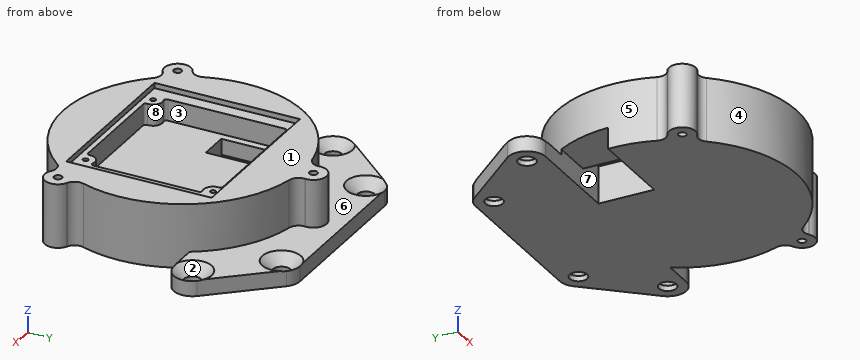
```python
from build123d import *

# Parameters (mm, degrees)
SKETCH_1_R                       = 22.554804791
EXTRUDE_463_DEPTH                = 6
SKETCH_2_W                       = 31.4
SKETCH_2_H                       = 27.4
CUT_EXTRUDE_592_DEPTH            = 5
SKETCH_3_R                       = 1.75
SKETCH_3_R_2                     = 0.5
EXTRUDE_810_DEPTH                = 4
SKETCH_4_W                       = 5.5
SKETCH_4_H                       = 10.5
USB_DEPTH                        = 33.28681524
SKETCH_5_W                       = 31.4
SKETCH_5_H                       = 27.4
SKETCH_5_W_2                     = 26.4
SKETCH_5_H_2                     = 25.4
EXTRUDE_1363_DEPTH               = 4
FILLET_1_R                       = 0.5
EXTRUDE_START                    = 6
SKETCH_6_R                       = 22.554804791
SKETCH_6_W                       = 5.5
SKETCH_6_H                       = 10.5
EXTRUDE_1904_DEPTH               = 6
SKETCH_7_W                       = 10.832625661
SKETCH_7_H                       = 10.5
CUT_EXTRUDE_2094_DEPTH           = 4
SKETCH_8_R                       = 1.65
EXTRUDE_2468_DEPTH               = 3
CHAMFER_1_SIZE                   = 2
EXTRUDE_START_2                  = -12
SKETCH_14_R                      = 0.75
EXTRUDE_2869_DEPTH               = 12
FILLET_3_R                       = 2
PATTERN_CIRCULAR_1_COUNT         = 3
FILLET_3_OF_PATTERN_CIRCULAR_1_R = 2


with BuildPart() as part:
    # Эскиз1 → Extrude 463 (new body)
    with BuildSketch(Plane.XY):
        Circle(SKETCH_1_R)
    extrude(amount=EXTRUDE_463_DEPTH)

    # Эскиз2 → Cut-Extrude 592 (cut)
    with BuildSketch(Plane.XY.offset(6)):
        Rectangle(SKETCH_2_W, SKETCH_2_H)
    extrude(amount=-CUT_EXTRUDE_592_DEPTH, mode=Mode.SUBTRACT)

    # Эскиз3 → Extrude 810 (add)
    # profile 1 of 3: a face of its own
    with BuildSketch(Plane.XY.offset(1)):
        with Locations((-12, -12)):
            Circle(SKETCH_3_R)
        with Locations((-12, -12)):
            Circle(SKETCH_3_R_2, mode=Mode.SUBTRACT)
    # profile 2 of 3: a face of its own
    with BuildSketch(Plane.XY.offset(1)):
        with Locations((12, -12)):
            Circle(SKETCH_3_R)
        with Locations((12, -12)):
            Circle(SKETCH_3_R_2, mode=Mode.SUBTRACT)
    # profile 3 of 3: a face of its own
    with BuildSketch(Plane.XY.offset(1)):
        with Locations((12, 12)):
            Circle(SKETCH_3_R)
        with Locations((12, 12)):
            Circle(SKETCH_3_R_2, mode=Mode.SUBTRACT)
    extrude(amount=EXTRUDE_810_DEPTH)

    # Эскиз4 → usb (cut, through all)
    with BuildSketch(Plane.XY.offset(1)):
        with Locations((-8.95, 6.25)):
            Rectangle(SKETCH_4_W, SKETCH_4_H)
    extrude(amount=-USB_DEPTH, mode=Mode.SUBTRACT)

    # Эскиз5 → Extrude 1363 (add)
    with BuildSketch(Plane.XY.offset(1)):
        Rectangle(SKETCH_5_W, SKETCH_5_H)
        Rectangle(SKETCH_5_W_2, SKETCH_5_H_2, mode=Mode.SUBTRACT)
    extrude(amount=EXTRUDE_1363_DEPTH)

    # Скругление1
    fillet_1_edges = [part.edges().sort_by_distance(p)[0] for p in [
        (10.396098507, 12.7, 3),
        (13.2, 10.72622608, 3),
        (10.396098507, -12.7, 3),
        (-13.2, -10.72622608, 3),
        (-10.396098507, -12.7, 3),
        (13.2, -10.72622608, 3),
        (-13.2, 12.7, 3),
    ]]
    fillet(fillet_1_edges, radius=FILLET_1_R)

    # Эскиз6 → Extrude 1904 (add)
    with BuildSketch(Plane(origin=(0, 0, 0), x_dir=(-1, 0, 0), z_dir=(0, 0, -1)).offset(EXTRUDE_START)):
        Circle(SKETCH_6_R)
        with Locations((8.95, 6.25)):
            Rectangle(SKETCH_6_W, SKETCH_6_H, mode=Mode.SUBTRACT)
    extrude(amount=-EXTRUDE_1904_DEPTH)

    # Эскиз7 → Cut-Extrude 2094 (cut)
    with BuildSketch(Plane(origin=(0, 0, -6), x_dir=(-1, 0, 0), z_dir=(0, 0, -1))):
        with Locations((17.116312831, 6.25)):
            Rectangle(SKETCH_7_W, SKETCH_7_H)
    extrude(amount=-CUT_EXTRUDE_2094_DEPTH, mode=Mode.SUBTRACT)

    # Эскиз8 → Extrude 2468 (add)
    with BuildSketch(Plane(origin=(0, 0, -6), x_dir=(-1, 0, 0), z_dir=(0, 0, -1))):
        with BuildLine():
            Line((-25, 11.5), (-19.402814723, 11.5))
            ThreePointArc((-19.402814723, 11.5), (0, 22.554804791), (19.402814723, 11.5))
            Line((19.402814723, 11.5), (25, 11.5))
            ThreePointArc((25, 11.5), (28.184979534, 13.548826209), (27.641119328, 17.296625502))
            Line((27.641119328, 17.296625502), (17.641119328, 28.796625502))
            ThreePointArc((17.641119328, 28.796625502), (16.451173791, 29.684979534), (15, 30))
            Line((15, 30), (-15, 30))
            ThreePointArc((-15, 30), (-16.451173791, 29.684979534), (-17.641119328, 28.796625502))
            Line((-17.641119328, 28.796625502), (-27.641119328, 17.296625502))
            ThreePointArc((-27.641119328, 17.296625502), (-28.184979534, 13.548826209), (-25, 11.5))
        make_face()
        with Locations((-15, 26.5)):
            Circle(SKETCH_8_R, mode=Mode.SUBTRACT)
        with Locations((15, 26.5)):
            Circle(SKETCH_8_R, mode=Mode.SUBTRACT)
        with Locations((25, 15)):
            Circle(SKETCH_8_R, mode=Mode.SUBTRACT)
        with Locations((-25, 15)):
            Circle(SKETCH_8_R, mode=Mode.SUBTRACT)
    extrude(amount=-EXTRUDE_2468_DEPTH)

    # Фаска1
    # the kernel refuses this chamfer: 2 mm, written as the material it takes off along each edge
    with BuildSketch(Plane(origin=(-25, 15, -3), x_dir=(-1, 0, 0), z_dir=(0, -1, 0))) as chamfer_1_piece_1:
        Polygon((1.65 + CHAMFER_1_SIZE, 0), (1.65, CHAMFER_1_SIZE), (1.65, 0), align=None)
    revolve(axis=Axis((-25, 15, -3), (0, 0, -1)), mode=Mode.SUBTRACT)
    with BuildSketch(Plane(origin=(-15, 26.5, -3), x_dir=(-1, 0, 0), z_dir=(0, -1, 0))) as chamfer_1_piece_2:
        Polygon((1.65 + CHAMFER_1_SIZE, 0), (1.65, CHAMFER_1_SIZE), (1.65, 0), align=None)
    revolve(axis=Axis((-15, 26.5, -3), (0, 0, -1)), mode=Mode.SUBTRACT)
    with BuildSketch(Plane(origin=(25, 15, -3), x_dir=(-1, 0, 0), z_dir=(0, -1, 0))) as chamfer_1_piece_3:
        Polygon((1.65 + CHAMFER_1_SIZE, 0), (1.65, CHAMFER_1_SIZE), (1.65, 0), align=None)
    revolve(axis=Axis((25, 15, -3), (0, 0, -1)), mode=Mode.SUBTRACT)
    with BuildSketch(Plane(origin=(15, 26.5, -3), x_dir=(-1, 0, 0), z_dir=(0, -1, 0))) as chamfer_1_piece_4:
        Polygon((1.65 + CHAMFER_1_SIZE, 0), (1.65, CHAMFER_1_SIZE), (1.65, 0), align=None)
    revolve(axis=Axis((15, 26.5, -3), (0, 0, -1)), mode=Mode.SUBTRACT)

    # Эскиз14 → Extrude 2869 (add)
    with BuildSketch(Plane.XY.offset(6).offset(EXTRUDE_START_2)):
        with BuildLine():
            Line((-22.403248133, -10.051512893), (-20.620019257, -9.139695017))
            ThreePointArc((-20.620019257, -9.139695017), (-19.533033926, -11.277402396), (-18.225217696, -13.287612994))
            Line((-18.225217696, -13.287612994), (-19.906489578, -14.376025564))
            ThreePointArc((-19.906489578, -14.376025564), (-23.430148244, -13.527402396), (-22.403248133, -10.051512893))
        make_face()
        with Locations((-21.265084734, -12.277402396)):
            Circle(SKETCH_14_R, mode=Mode.SUBTRACT)
    extrude_2869 = extrude(amount=EXTRUDE_2869_DEPTH)

    # Скругление3
    fillet_3_edges = [part.edges().sort_by_distance(p)[0] for p in [
        (-20.620019257, -9.139695017, 0),
        (-18.225217696, -13.287612994, 0),
    ]]
    fillet(fillet_3_edges, radius=FILLET_3_R)

    # Круговой массив1: Extrude 2869 ×3 about axis
    pattern_circular_1_axis = Axis((0, 0, 0), (0, 0, 1))
    for i in range(1, PATTERN_CIRCULAR_1_COUNT):
        add(extrude_2869.rotate(pattern_circular_1_axis, i * 360 / PATTERN_CIRCULAR_1_COUNT))

    # Скругление3 of Круговой массив1
    fillet_3_of_pattern_circular_1_edges = [part.edges().sort_by_distance(p)[0] for p in [
        (18.225217696, -13.287612994, 0),
        (20.620019257, -9.139695017, 0),
        (2.394801561, 22.427308012, 0),
        (-2.394801561, 22.427308012, 0),
    ]]
    fillet(fillet_3_of_pattern_circular_1_edges, radius=FILLET_3_OF_PATTERN_CIRCULAR_1_R)


solid = part.part
```
Verification items for the finished model (mm, model axes). Face numbers are marked on the shaded views. A direction names the side the tool comes from. Coordinates: 2 decimals unless noted, no trailing zeros. Order: outer loops, then holes, each group sorted by start corner. A loop starts at its lowest first (then second) coordinate and runs counter-clockwise, first axis right, second up. Notation, with made-up numbers: (30, -9) - (67, -9) arc R21 ccw to (67, 30) - close; hole circle Ø11 at (-14.75, 76.5). An arc over 180 degrees is marked (long way). Return JSON: item names as keys, results as strings.
(1) Access from +Z, -Z, +X, -X, +Y, -Y to the whole of each face (thin tool, end or side, straight path). Record for the marked faces 5, 6, 7 and 8.
Filled sheet:
{"face 5": "+Z, -X", "face 6": "+Z, +Y", "face 7": "-Z", "face 8": "+Z"}
(2) Section check B-B, the plane z = 0. Give the number of separate pieces and of enclosed holes in the cut face, and give its area (3 significant figures).
Filled sheet:
{"separate pieces": "1", "enclosed holes": "4", "area": "1,600 mm^2"}
(3) Mould release check, pull along Y, two halves, no side actions. Record for the marked faces 1, 2, 3 and 4: pulls with the +Y half, pulls with the -Y half, needs draft (parallel to the pull), parting line crosses it, or undercut.
Filled sheet:
{"face 1": "needs draft", "face 2": "undercut", "face 3": "undercut", "face 4": "pulls with the -Y half"}
(4) Section check D-D, the plane y = 21.5. Record the cut outline in (x, z).
Filled sheet:
{"outline": "(-23.99, -6) - (23.99, -6) - (23.99, -3) - (6.82, -3) - (6.82, 6) - (-6.82, 6) - (-6.82, -3) - (-23.99, -3) - close"}
(5) Section check A-A, the plane y = 15. Record the cut outline in (x, z).
Filled sheet:
{"outline": "(-28.5, -6) - (-26.65, -6) - (-26.65, -5) - (-28.5, -3.15) - close; (-23.35, -6) - (23.35, -6) - (23.35, -5) - (21.35, -3) - (16.84, -3) - (16.84, 6) - (-16.84, 6) - (-16.84, -3) - (-21.35, -3) - (-23.35, -5) - close; (26.65, -6) - (28.5, -6) - (28.5, -3.15) - (26.65, -5) - close"}
(6) Go/stop test with flat-tipped pins: pin 1 (5.5 mm diameter, centred on y = 6, z = -4, fed in from -X); pin 2 (0.8 mm diameter, centred on x = 12, y = 12, fed in from +Z); pin 3 (5 mm diameter, centred on x = -16, z = 4.5, fed in from -Y). Record where each tip stops, or that it passes through.
Filled sheet:
{"pin 1": "stops at x = -22.18", "pin 2": "stops at z = 1", "pin 3": "stops at y = -18.07"}
(7) Thickness scan on line 1 along Y through (x, z) = (23.5, -3.25); line 2 along Z through (x, y) = (-11, 20); line 3 along Z through (x, y) = (-1.5, 5). Record the ranges inside material, lowest first.
Filled sheet:
{"line 1": "y = -13.4 to -11.16, 11.5 to 11.95, 18.05 to 22.06", "line 2": "z = -6 to -3", "line 3": "z = -6 to 1"}
